CAD build for the part. Positions are in the model's coordinates, mm. A direction names the side the tool comes from. Coordinates: 2 decimals unless noted, no trailing zeros. Order: outer loops, then holes, each group sorted by start corner. A loop starts at its lowest first (then second) coordinate and runs counter-clockwise, first axis right, second up. Notation, with made-up numbers: (65, 89) - (84, 89) arc R15 cw to (84, 107) - close; hole circle Ø4 at (70, 34). An arc over 180 degrees is marked (long way). Return JSON: item names as keys, results as strings.
from build123d import *


with BuildPart() as f1:
    # F0 (on Right) → F1 (revolve)
    with BuildSketch(Plane.YZ):
        with BuildLine():
            Line((21.45, 3), (16.45, 3))
            ThreePointArc((16.45, 3), (15.7428932188, 2.7071067812), (15.45, 2))
            Line((15.45, 2), (15.45, 1))
            ThreePointArc((15.45, 1), (15.7428932188, 0.2928932188), (16.45, 0))
            Line((16.45, 0), (17.45, 0))
            Line((17.45, 0), (17.45, -19))
            ThreePointArc((17.45, -19), (17.7428932188, -19.7071067812), (18.45, -20))
            Line((18.45, -20), (21.45, -20))
            ThreePointArc((21.45, -20), (22.1571067812, -19.7071067812), (22.45, -19))
            Line((22.45, -19), (22.45, 2))
            ThreePointArc((22.45, 2), (22.1571067812, 2.7071067812), (21.45, 3))
        make_face()
    revolve(axis=Axis((0, 0, -3.255167976), (0, 0, -1)))


solid = f1.part
Item 1: Wall check: L1, parallel to X at y = 0, z = -4; L2, parallel to Y at x = -5.5, z = -8.25; L3, parallel to Y at x = 15, z = -10.25. Give the ranges that are in metal, low to high. Write a range as [from, to].
Findings below:
{"L1": "x = [-22.45, -17.45], [17.45, 22.45]", "L2": "y = [-21.77, -16.56], [16.56, 21.77]", "L3": "y = [-16.7, -8.92], [8.92, 16.7]"}
Item 2: Drop flat-ended pins along their axis: P1, Ø10, axis at x = 12, z = -13, coming from the -Y side; P2, Ø12, axis at x = 16, z = -1, coming from the +Y side; P3, Ø8, axis at y = 2, z = -11.5, coming from the -X side. Give the stop position or say it passes through.
Findings below:
{"P1": "stops at y = -21.33", "P2": "stops at y = 20.1", "P3": "stops at x = -22.45"}
Item 3: Which spindle directions (+Z, -Z, +X, -X, +Y, -Y) get a long thin tool onto all of the face, cutting with end or side? Do faces 4 (the flat face through (16, 5, 0)), 5 (the cylindrical face through (-9.4, -12.26, 1.49)). Say none if no direction does.
Findings below:
{"face 4": "-Z", "face 5": "+Z, -Z"}
Item 4: Band-saw the part on C-C, the plane z = -17.75. List the corners of the cut face in (x, y).
Findings below:
{"outline": "circle Ø44.9 at (0, 0); hole circle Ø34.9 at (0, 0)"}
Item 5: Mould opens along X. For faces 1 (the cylindrical face through (-17.035, -3.783, -9.633)), 2 (the flat face through (-16, -5, 3)), 3 (the cylindrical face through (15.17, -16.55, -8.35)) say: released by +X, released by -X, zero draft, split by the parting line, or undercut.
Findings below:
{"face 1": "undercut", "face 2": "zero draft", "face 3": "split by the parting line"}
Item 6: Band-saw the part on A-A, the plane y = 0. List the corners of the cut face in (x, z).
Findings below:
{"outline": "(-22.45, -19) arc R1 ccw to (-21.45, -20) - (-18.45, -20) arc R1 ccw to (-17.45, -19) - (-17.45, 0) - (-16.45, 0) arc R1 ccw to (-15.45, 1) - (-15.45, 2) arc R1 ccw to (-16.45, 3) - (-21.45, 3) arc R1 ccw to (-22.45, 2) - close; (15.45, 1) arc R1 ccw to (16.45, 0) - (17.45, 0) - (17.45, -19) arc R1 ccw to (18.45, -20) - (21.45, -20) arc R1 ccw to (22.45, -19) - (22.45, 2) arc R1 ccw to (21.45, 3) - (16.45, 3) arc R1 ccw to (15.45, 2) - close"}
